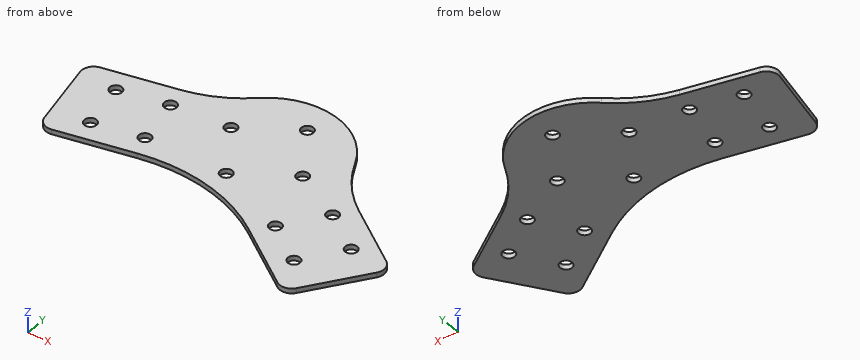
```python
from build123d import *

# Parameters (mm, degrees)
SKETCH1_R           = 2.5
BOSS_EXTRUDE1_DEPTH = 2
FILLET1_R           = 50
FILLET2_R           = 70
FILLET3_R           = 5


with BuildPart() as part:
    # Sketch1 → Boss-Extrude1 (new body)
    with BuildSketch(Plane.XY):
        with BuildLine():
            Line((-77.311392181, 2.991427603), (-69.410747929, -34.178181225))
            Line((-69.410747929, -34.178181225), (-4.13058082, -20.302453359))
            Line((-4.13058082, -20.302453359), (50.538451031, -58.582121568))
            Line((50.538451031, -58.582121568), (72.334355612, -27.454343885))
            Line((72.334355612, -27.454343885), (29.915692131, 2.247524046))
            ThreePointArc((29.915692131, 2.247524046), (5.981038033, 29.397741139), (-26.659362194, 13.757848938))
            Line((-26.659362194, 13.757848938), (-77.311392181, 2.991427603))
        make_face()
        with Locations((-60.767972952, -2.693225442)):
            Circle(SKETCH1_R, mode=Mode.SUBTRACT)
        with Locations(Location((-56.609739136, -22.256177456, 0), (0, 0, 180))):
            Circle(SKETCH1_R, mode=Mode.SUBTRACT)
        with Locations((-37.046787121, -18.09794364)):
            Circle(SKETCH1_R, mode=Mode.SUBTRACT)
        with Locations(Location((-41.205020938, 1.465008375, 0), (0, 0, 180))):
            Circle(SKETCH1_R, mode=Mode.SUBTRACT)
        with Locations((38.501846135, -14.751537011)):
            Circle(SKETCH1_R, mode=Mode.SUBTRACT)
        with Locations(Location((27.030317408, -31.134577897, 0), (0, 0, 180))):
            Circle(SKETCH1_R, mode=Mode.SUBTRACT)
        with Locations((43.413358294, -42.606106624)):
            Circle(SKETCH1_R, mode=Mode.SUBTRACT)
        with Locations(Location((54.884887021, -26.223065738, 0), (0, 0, 180))):
            Circle(SKETCH1_R, mode=Mode.SUBTRACT)
        with Locations((3.58862282, 17.638644683)):
            Circle(SKETCH1_R, mode=Mode.SUBTRACT)
        with Locations((17.638644683, -3.58862282)):
            Circle(SKETCH1_R, mode=Mode.SUBTRACT)
        with Locations((-3.58862282, -17.638644683)):
            Circle(SKETCH1_R, mode=Mode.SUBTRACT)
        with Locations((-17.638644683, 3.58862282)):
            Circle(SKETCH1_R, mode=Mode.SUBTRACT)
    extrude(amount=BOSS_EXTRUDE1_DEPTH)

    # Fillet1
    fillet1_edges = [part.edges().sort_by_distance(p)[0] for p in [
        (-26.659362194, 13.757848938, 1),
        (29.915692131, 2.247524046, 1),
    ]]
    fillet(fillet1_edges, radius=FILLET1_R)

    # Fillet2
    fillet2_edges = [part.edges().sort_by_distance(p)[0] for p in [
        (-4.13058082, -20.302453359, 1),
    ]]
    fillet(fillet2_edges, radius=FILLET2_R)

    # Fillet3
    fillet3_edges = [part.edges().sort_by_distance(p)[0] for p in [
        (72.334355612, -27.454343885, 1),
        (50.538451031, -58.582121568, 1),
        (-69.410747929, -34.178181225, 1),
        (-77.311392181, 2.991427603, 1),
    ]]
    fillet(fillet3_edges, radius=FILLET3_R)


solid = part.part
```
Geometry: final body of the model. Coordinates: model frame, mm. Round coordinates to 2 decimals unless told otherwise and drop trailing zeros. Write each loop counter-clockwise with the first axis right and the second up, starting at its lowest first coordinate (ties: lowest second). Pieces come first, ordered by that corner, then holes. Notation, with made-up numbers: (-27.75, 15) -> (28.25, 15) arc R24 cw to (28.25, 26) -> close; hole circle Ø8 at (-39, 30.5). An arc over 180 degrees is marked (long way). Return JSON: item names as keys, results as strings.
Q1. First-contact query: pin 1 Ø4.5 at (x, y) = (-3.59, -17.64) entering from +Z; pin 2 Ø6.5 at (x, y) = (43.41, -42.61) entering from -Z; pin 3 Ø1 at (x, z) = (29.5, 1) entering from +Y. Flat tips, straight axial feed; report the tip coordinate or a pass-through.
From the geometry:
{"pin 1": "through", "pin 2": "z = 0", "pin 3": "y = 9.08"}
Q2. Section B-B on z = 0.6. Give the number of separate pieces and of enclosed holes in the cut face, and give its area (3 significant figures).
From the geometry:
{"separate pieces": "1", "enclosed holes": "12", "area": "6,180 mm2"}
Q3. Section A-A on x = -17. Return the cut outline in (y, z).
From the geometry:
{"outline": "(-25.14, 0) -> (1.17, 0) -> (1.17, 2) -> (-25.14, 2) -> close; (6.01, 0) -> (24.72, 0) -> (24.72, 2) -> (6.01, 2) -> close"}
Q4. Ray query, line 1 (X direction, y = -3, z = 1.35); line 2 (X direction, y = -4, z = 1.4); line 3 (Y direction, x = 18, z = 0.2). Return the intervals inside material, ascending.
From the geometry:
{"line 1": "-76.04 to -63.25, -58.29 to 15.21, 20.07 to 38.36", "line 2": "-75.83 to -62.9, -58.64 to 15.17, 20.1 to 39.44", "line 3": "-35.9 to -6.06, -1.11 to 24"}
Q5. Section C-C on x = 12.5. Return the cut outline in (y, z), and give its area (3 significant figures).
From the geometry:
{"outline": "(-32.77, 0) -> (27.27, 0) -> (27.27, 2) -> (-32.77, 2) -> close", "area": "120 mm2"}
